```python
from build123d import *

# Parameters (mm, degrees)
F1_DEPTH = 2.54
F2_R     = 3.080736
F2_R_2   = 1.935305
F3_DEPTH = 3.81


with BuildPart() as f1:
    # F0 (on Front) → F1 (new body)
    with BuildSketch(Plane.XZ):
        Polygon((12.7, -10.405478), (12.7, -2.785478), (-12.7, -2.785478), (-12.7, -10.405478), (0, -10.405478), align=None)
    extrude(amount=F1_DEPTH)

    # F2 (on face) → F3 (join)
    with BuildSketch(Plane(origin=(0, 0, 0), x_dir=(-1, 0, 0), z_dir=(0, 1, 0))):
        with Locations((-7.207552, -6.461604)):
            Circle(F2_R)
        with Locations((-7.207552, -6.461604)):
            Circle(F2_R_2, mode=Mode.SUBTRACT)
        with Locations((7.207552, -6.461604)):
            Circle(F2_R)
        with Locations((7.207552, -6.461604)):
            Circle(F2_R_2, mode=Mode.SUBTRACT)
    extrude(amount=F3_DEPTH)


solid = f1.part
```
Build history of the part. All positions in model axes, mm. A direction names the side the tool comes from. Give positions to 0.01 mm unless a question says otherwise; leave off trailing zeros. Loops run counter-clockwise (first coordinate to the right, second up) from the corner with the lowest first, then second, coordinate; pieces in that order, holes last. Notation, with made-up numbers: (77.25, -7.5) -> (96.25, -7.5) arc R33 cw to (96.25, 22.5) -> close; hole circle Ø10 at (43, 42.25). An arc over 180 degrees is marked (long way). One line per question, with ' | ' between items. Start each with the question number.
1) Cut at D-D (x = -10). Give the cut face in (y, z), plus the area to 3 significant figures.
2) 3-axis set-ups, long thin cutter, end or side, ignore diameter. For faces 1 (the flat face through (12.7, -1, -7)), 2 (the flat face through (-7, 0, -6)): which of +Z, -Z, +X, -X, +Y, -Y reach the whole face in a straight line?
3) Pin check, flat tips, straight feed: pin 1 (3 mm diameter, centred on x = 0, z = -4, fed in from +Y); pin 2 (1.5 mm diameter, centred on x = -8, y = 3, fed in from -Z). Stop position of each tip, or through.
4) Two-plate mould, pull along X, no slides. Class faces 3 (the flat face through (-12.7, -1, -7)), 4 (the flat face through (0, -1, -2.785)), 5 (the cylindrical face through (9.48, 1.88, -4.38)): released by +X, released by -X, zero draft, split by the parting line, or undercut.
5) Cut at A-A (x = 8). Give the cut face in (y, z), plus the area to 3 significant figures.
6) Cut at C-C (y = 0.5). Give the cut face in (x, z).
7) Cut at B-B (z = -8). Give the cut face in (x, y), plus the area to 3 significant figures.
8) Probe L1, parallel to X at y = 3.25, z = -6.5; L2, parallel to X at y = 1.25, z = -5.25; L3, parallel to Y at x = 11.5, z = -7.25. List the from-to ranges inside material, lowest first.
Return value:
1) outline: (-2.54, -10.41) -> (0, -10.41) -> (0, -7.76) -> (3.81, -7.76) -> (3.81, -5.16) -> (0, -5.16) -> (0, -2.79) -> (-2.54, -2.79) -> close | area: 29.3 mm^2
2) face 1: +Z, -Z, +X, +Y, -Y | face 2: +Y
3) pin 1: y = 0 | pin 2: z = -9.54
4) face 3: released by -X | face 4: zero draft | face 5: undercut
5) outline: (-2.54, -10.41) -> (0, -10.41) -> (0, -9.44) -> (3.81, -9.44) -> (3.81, -8.23) -> (0, -8.23) -> (0, -4.7) -> (3.81, -4.7) -> (3.81, -3.48) -> (0, -3.48) -> (0, -2.79) -> (-2.54, -2.79) -> close | area: 28.6 mm^2
6) outline: circle Ø6.16 at (-7.21, -6.46); circle Ø6.16 at (7.21, -6.46); hole circle Ø3.87 at (-7.21, -6.46); hole circle Ø3.87 at (7.21, -6.46)
7) outline: (-12.7, -2.54) -> (12.7, -2.54) -> (12.7, 0) -> (9.88, 0) -> (9.88, 3.81) -> (8.38, 3.81) -> (8.38, 0) -> (6.03, 0) -> (6.03, 3.81) -> (4.54, 3.81) -> (4.54, 0) -> (-4.54, 0) -> (-4.54, 3.81) -> (-6.03, 3.81) -> (-6.03, 0) -> (-8.38, 0) -> (-8.38, 3.81) -> (-9.88, 3.81) -> (-9.88, 0) -> (-12.7, 0) -> close | area: 87.3 mm^2
8) L1: -10.29 to -9.14, -5.27 to -4.13, 4.13 to 5.27, 9.14 to 10.29 | L2: -10.04 to -8.72, -5.7 to -4.38, 4.38 to 5.7, 8.72 to 10.04 | L3: -2.54 to 0
